```python
from build123d import *

# Parameters (mm, degrees)
SKETCH_1_R      = 1.5
EXTRUDE_1_DEPTH = 2


with BuildPart() as part:
    # 草图1 → 凸台-拉伸1 (new body)
    with BuildSketch(Plane(origin=(0, 0, 0), x_dir=(1, 0, 0), z_dir=(0, 1, 0))):
        with BuildLine():
            Line((-5.6, 6.9), (-5.6, 13))
            ThreePointArc((-5.6, 13), (-6.185786438, 14.414213562), (-7.6, 15))
            Line((-7.6, 15), (-39.2, 15))
            ThreePointArc((-39.2, 15), (-40.614213562, 14.414213562), (-41.2, 13))
            Line((-41.2, 13), (-41.2, -13))
            ThreePointArc((-41.2, -13), (-40.614213562, -14.414213562), (-39.2, -15))
            Line((-39.2, -15), (-7.6, -15))
            ThreePointArc((-7.6, -15), (-6.185786438, -14.414213562), (-5.6, -13))
            Line((-5.6, -13), (-5.6, -6.9))
            Line((-5.6, -6.9), (5.6, -6.9))
            Line((5.6, -6.9), (5.6, -13))
            ThreePointArc((5.6, -13), (6.185786438, -14.414213562), (7.6, -15))
            Line((7.6, -15), (39.2, -15))
            ThreePointArc((39.2, -15), (40.614213562, -14.414213562), (41.2, -13))
            Line((41.2, -13), (41.2, 13))
            ThreePointArc((41.2, 13), (40.614213562, 14.414213562), (39.2, 15))
            Line((39.2, 15), (7.6, 15))
            ThreePointArc((7.6, 15), (6.185786438, 14.414213562), (5.6, 13))
            Line((5.6, 13), (5.6, 6.9))
            Line((5.6, 6.9), (-5.6, 6.9))
        make_face()
        with Locations(Location((-20, -11.75, 0), (0, 0, 270))):
            Circle(SKETCH_1_R, mode=Mode.SUBTRACT)
        with Locations(Location((20, -11.75, 0), (0, 0, 270))):
            Circle(SKETCH_1_R, mode=Mode.SUBTRACT)
        with Locations(Location((20, 11.75, 0), (0, 0, 90))):
            Circle(SKETCH_1_R, mode=Mode.SUBTRACT)
        with Locations(Location((-20, 11.75, 0), (0, 0, 90))):
            Circle(SKETCH_1_R, mode=Mode.SUBTRACT)
        with Locations(Location((-29.3, 0, 0), (0, 0, 270))):
            Circle(SKETCH_1_R, mode=Mode.SUBTRACT)
        with Locations(Location((29.3, 0, 0), (0, 0, 270))):
            Circle(SKETCH_1_R, mode=Mode.SUBTRACT)
        with BuildLine():
            Line((33.225, 5), (33.225, -5))
            ThreePointArc((33.225, -5), (32.6, -5.625), (31.975, -5))
            Line((31.975, -5), (31.975, 5))
            ThreePointArc((31.975, 5), (32.6, 5.625), (33.225, 5))
        make_face(mode=Mode.SUBTRACT)
        with BuildLine():
            Line((37.225, 5), (37.225, -5))
            ThreePointArc((37.225, -5), (36.6, -5.625), (35.975, -5))
            Line((35.975, -5), (35.975, 5))
            ThreePointArc((35.975, 5), (36.6, 5.625), (37.225, 5))
        make_face(mode=Mode.SUBTRACT)
        with BuildLine():
            Line((-37.225, 5), (-37.225, -5))
            ThreePointArc((-37.225, -5), (-36.6, -5.625), (-35.975, -5))
            Line((-35.975, -5), (-35.975, 5))
            ThreePointArc((-35.975, 5), (-36.6, 5.625), (-37.225, 5))
        make_face(mode=Mode.SUBTRACT)
        with BuildLine():
            Line((-33.225, 5), (-33.225, -5))
            ThreePointArc((-33.225, -5), (-32.6, -5.625), (-31.975, -5))
            Line((-31.975, -5), (-31.975, 5))
            ThreePointArc((-31.975, 5), (-32.6, 5.625), (-33.225, 5))
        make_face(mode=Mode.SUBTRACT)
    extrude(amount=EXTRUDE_1_DEPTH)


solid = part.part
```
CAD build for the part. Positions are in the model's coordinates, mm. A direction names the side the tool comes from. Coordinates: 2 decimals unless noted, no trailing zeros. Order: outer loops, then holes, each group sorted by start corner. A loop starts at its lowest first (then second) coordinate and runs counter-clockwise, first axis right, second up. Notation, with made-up numbers: (26, 69) -> (50, 69) arc R15 cw to (50, 87) -> close; hole circle Ø11 at (60.5, 58). An arc over 180 degrees is marked (long way). Use one line per item in the form item = value. Start each with the question number.
1) Band-saw the part on D-D on z = 12.25. Give the cut face in (x, y).
2) Tool access for faces 1 (the cylindrical face through (6.17, 0.99, 14.4)), 2 (the flat face through (-35.975, 1, 0)), 3 (the flat face through (0, 1, -6.9)): list every direction of +Z, -Z, +X, -X, +Y, -Y with a clear straight run to the whole face (end or side of a thin tool).
3) Band-saw the part on A-A on x = -29.3. Give the cut face in (y, z).
4) Pull direction X, two halves, no side cores. Call faces 4 (the flat face through (-23, 1, -15)), 5 (the cylindrical face through (-40.6, 0.99, -14.43)), 6 (the flat face through (-5.6, 1, 10)): +X half, -X half, draft (parallel to the pull), parting line (faces both ways), or undercut.
5) Band-saw the part on C-C on x = -20. Give the cut face in (y, z), then the cut area to 3 significant figures.
6) Drill centre lines: L1, parallel to X at y = 0.35, z = 3.5 (3 decimals); L2, parallel to X at y = 0.7, z = 11.75; L3, parallel to Z at x = -21, y = 1.75. Where is each one in solid material? Low to high. Write a range as [from, to].
7) Band-saw the part on B-B on z = 0. Give the cut face in (x, y) (3 decimals).
Entries:
q1.outline = (-41.2, 0) -> (-21.41, 0) -> (-21.41, 2) -> (-41.2, 2) -> close; (-18.59, 0) -> (-5.6, 0) -> (-5.6, 2) -> (-18.59, 2) -> close; (5.6, 0) -> (18.59, 0) -> (18.59, 2) -> (5.6, 2) -> close; (21.41, 0) -> (41.2, 0) -> (41.2, 2) -> (21.41, 2) -> close
q2.face_1 = +Z, +Y, -Y
q2.face_2 = +Y, -Y
q2.face_3 = -Z, +Y, -Y
q3.outline = (0, -15) -> (2, -15) -> (2, -1.5) -> (0, -1.5) -> close; (0, 1.5) -> (2, 1.5) -> (2, 15) -> (0, 15) -> close
q4.face_4 = draft
q4.face_5 = -X half
q4.face_6 = undercut
q5.outline = (0, -15) -> (2, -15) -> (2, -13.25) -> (0, -13.25) -> close; (0, -10.25) -> (2, -10.25) -> (2, 10.25) -> (0, 10.25) -> close; (0, 13.25) -> (2, 13.25) -> (2, 15) -> (0, 15) -> close
q5.area = 48.0 mm2
q6.L1 = [-41.2, -37.225], [-35.975, -33.225], [-31.975, 31.975], [33.225, 35.975], [37.225, 41.2]
q6.L2 = [-41.2, -21.5], [-18.5, -5.6], [5.6, 18.5], [21.5, 41.2]
q6.L3 = [-15, -12.87], [-10.63, 10.63], [12.87, 15]
q7.outline = (-41.2, 0) -> (-37.225, 0) -> (-37.225, 2) -> (-41.2, 2) -> close; (-35.975, 0) -> (-33.225, 0) -> (-33.225, 2) -> (-35.975, 2) -> close; (-31.975, 0) -> (-30.8, 0) -> (-30.8, 2) -> (-31.975, 2) -> close; (-27.8, 0) -> (27.8, 0) -> (27.8, 2) -> (-27.8, 2) -> close; (30.8, 0) -> (31.975, 0) -> (31.975, 2) -> (30.8, 2) -> close; (33.225, 0) -> (35.975, 0) -> (35.975, 2) -> (33.225, 2) -> close; (37.225, 0) -> (41.2, 0) -> (41.2, 2) -> (37.225, 2) -> close
